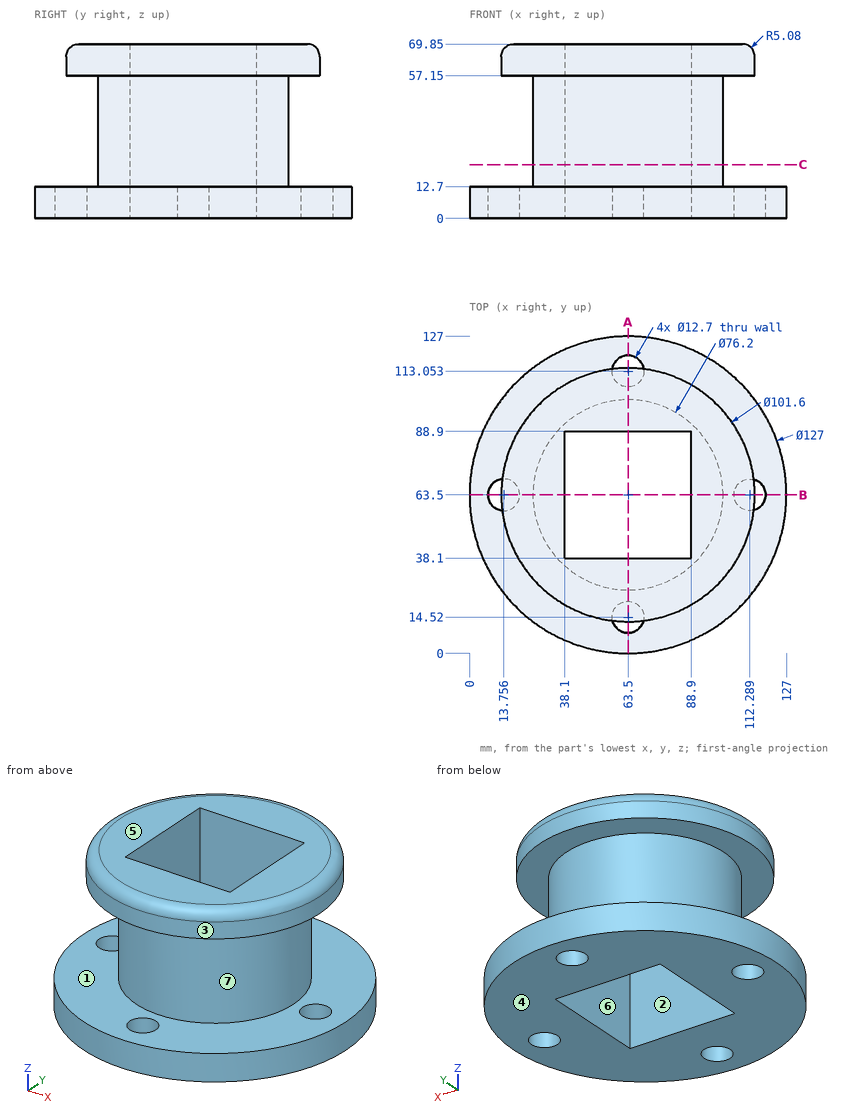
Source: three-view drawing plus pictorial views. Frame: mm from the lowest corner of the part. A direction names the side the tool comes from. Coordinates: 2 decimals unless noted, no trailing zeros. Order: outer loops, then holes, each group sorted by start corner. A loop starts at its lowest first (then second) coordinate and runs counter-clockwise, first axis right, second up. Notation, with made-up numbers: M 27.25,-7.5 L 48.25,-7.5 A27 cw 48.25,21.5 Z; hole C -14,63 d3. An arc over 180 degrees is marked long. Answer in a Markdown table with one row per item.
(1) Section query A-A, the plane x = 63.5. Output: boundary loops of the cut face in (y, z).
Numbers:
| item | result |
|---|---|
| outline | M 0,0 L 8.17,0 L 8.17,12.7 L 0,12.7 Z; M 12.7,57.15 L 25.4,57.15 L 25.4,12.7 L 20.87,12.7 L 20.87,0 L 38.1,0 L 38.1,69.85 L 17.78,69.85 A5.08 ccw 12.7,64.77 Z; M 88.9,0 L 106.7,0 L 106.7,12.7 L 101.6,12.7 L 101.6,57.15 L 114.3,57.15 L 114.3,64.77 A5.08 ccw 109.22,69.85 L 88.9,69.85 Z; M 119.4,0 L 127,0 L 127,12.7 L 119.4,12.7 Z |
(2) Contact query for flat-ended pins moving along their axis: pin 1 Ø15 at (y, z) = (70.5, 29) entering from +X; pin 2 Ø10 at (x, z) = (83, 42.5) entering from -Y; pin 3 Ø1 at (y, z) = (66, 56.5) entering from -X. Output: stop coordinate, or through.
Numbers:
| item | result |
|---|---|
| pin 1 | stops at x = 101.6 |
| pin 2 | stops at y = 28.27 |
| pin 3 | stops at x = 25.45 |
(3) Material intervals for line 1 (Y direction, x = 63.5, z = 7); line 2 (X direction, y = 63, z = 8); line 3 (Z direction, x = 21, y = 67.5), sorted ascending. Write a range as [from, to].
Numbers:
| item | result |
|---|---|
| line 1 | y = [0, 8.17], [20.87, 38.1], [88.9, 106.7], [119.4, 127] |
| line 2 | x = [0, 7.43], [20.09, 38.1], [88.9, 105.96], [118.62, 127] |
| line 3 | z = [0, 12.7], [57.15, 69.85] |
(4) Access query for the marked faces 1, 2, 3 and 4. Directions: +Z, -Z, +X, -X, +Y, -Y. A direction counts if a zero-diameter tool reaches every point of the face in a straight line with its end or side. Return the directions, or none.
Numbers:
| item | result |
|---|---|
| face 1 | none |
| face 2 | +Z, -Z |
| face 3 | +Z |
| face 4 | -Z, +X, -X, +Y, -Y |
(5) Draft query along Y for the marked faces 5, 6 and 7. Return one class per face: pulls with the +Y half, pulls with the -Y half, needs draft (parallel to the pull), parting line crosses it, or undercut.
Numbers:
| item | result |
|---|---|
| face 5 | needs draft |
| face 6 | undercut |
| face 7 | parting line crosses it |
(6) Section query C-C, the plane z = 21.5. Output: boundary loops of the cut face in (x, y).
Numbers:
| item | result |
|---|---|
| outline | C 63.5,63.5 d76.2; hole M 38.1,38.1 L 88.9,38.1 L 88.9,88.9 L 38.1,88.9 Z |
(7) Section query B-B, the plane y = 63.5. Output: boundary loops of the cut face in (x, z), plus the area to 3 significant figures.
Numbers:
| item | result |
|---|---|
| outline | M 0,0 L 7.41,0 L 7.41,12.7 L 0,12.7 Z; M 12.7,57.15 L 25.4,57.15 L 25.4,12.7 L 20.11,12.7 L 20.11,0 L 38.1,0 L 38.1,69.85 L 17.78,69.85 A5.08 ccw 12.7,64.77 Z; M 88.9,0 L 105.94,0 L 105.94,12.7 L 101.6,12.7 L 101.6,57.15 L 114.3,57.15 L 114.3,64.77 A5.08 ccw 109.22,69.85 L 88.9,69.85 Z; M 118.64,0 L 127,0 L 127,12.7 L 118.64,12.7 Z |
| area | 2,410 mm^2 |
